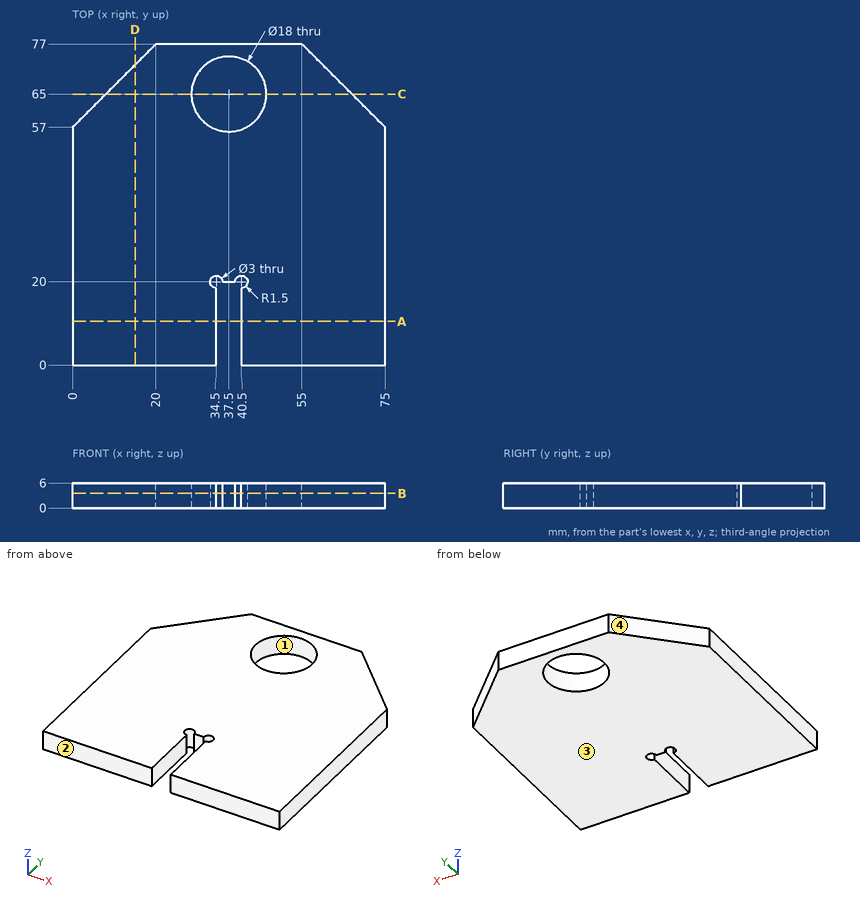
Geometry: see drawing. Coordinates: mm, zero at the bounding-box minimum. Coordinates: 2 decimals unless noted, no trailing zeros. Loops run counter-clockwise (first coordinate to the right, second up) from the corner with the lowest first, then second, coordinate; pieces in that order, holes last. Notation, with made-up numbers: (13.5, -21.5) -> (43.5, -21.5) arc R32 cw to (43.5, 11.5) -> close; hole circle Ø7 at (85, 54.5). An arc over 180 degrees is marked (long way). Use a Markdown table: item, result.
1) Material intervals for line 1 along X through (y, z) = (5, 3.1); line 2 along Y through (x, z) = (35, 4.2); line 3 along Y through (x, z) = (39.5, 4.2) (1 decimal), sorted ascending. Write a range as from..to.
Results found:
| item | result |
|---|---|
| line 1 | x = 0..34.5, 40.5..75 |
| line 2 | y = 21.41..56.35, 73.65..77 |
| line 3 | y = 21.1..56.2, 73.8..77 |
2) Pull-direction query (Y, two-part tool) for the marked faces 1, 2, 3 and 4; classes: released by +Y, released by -Y, zero draft, split by the parting line, or undercut.
Results found:
| item | result |
|---|---|
| face 1 | undercut |
| face 2 | released by -Y |
| face 3 | zero draft |
| face 4 | released by +Y |
3) Contact query for flat-ended pins moving along their axis: pin 1 (0.9 mm diameter, centred on x = 37, z = 2, fed in from -Y); pin 2 (1 mm diameter, centred on y = 66, z = 1.5, fed in from -X). Output: stop coordinate, or through.
Results found:
| item | result |
|---|---|
| pin 1 | stops at y = 20 |
| pin 2 | stops at x = 8.5 |
4) Cut plane C-C (y = 65). Return the cut outline in (x, z), then the cut area to 3 significant figures.
Results found:
| item | result |
|---|---|
| outline | (8, 0) -> (28.5, 0) -> (28.5, 6) -> (8, 6) -> close; (46.5, 0) -> (67, 0) -> (67, 6) -> (46.5, 6) -> close |
| area | 246 mm2 |
5) Cut plane D-D (x = 15). Return the cut outline in (y, z).
Results found:
| item | result |
|---|---|
| outline | (0, 0) -> (72, 0) -> (72, 6) -> (0, 6) -> close |
6) Cut plane A-A (y = 10.5). Return the cut outline in (x, z).
Results found:
| item | result |
|---|---|
| outline | (0, 0) -> (34.5, 0) -> (34.5, 6) -> (0, 6) -> close; (40.5, 0) -> (75, 0) -> (75, 6) -> (40.5, 6) -> close |
7) Cut plane B-B (z = 3.55). Return the cut outline in (x, y).
Results found:
| item | result |
|---|---|
| outline | (0, 0) -> (34.5, 0) -> (34.5, 18.5) arc R1.5 cw (long way) to (36, 20) -> (39, 20) arc R1.5 cw (long way) to (40.5, 18.5) -> (40.5, 0) -> (75, 0) -> (75, 57) -> (55, 77) -> (20, 77) -> (0, 57) -> close; hole circle Ø18 at (37.5, 65) |
